```python
from build123d import *

# Parameters (mm, degrees)
F1_DEPTH    = 2
F3_DEPTH    = 13
F2_W        = 100
F2_H        = 2
F4_DEPTH    = 25
F5_W        = 1.9823738266
F5_H        = 13
F6_DEPTH    = 6
F7_T1_DEPTH = 18.1433659759
F9_DEPTH    = 25


# Not quite as in the source:
# - a fillet or chamfer that OpenCascade refuses, or shapes differently, is made with other operations: its cross-section is extruded or revolved along the edge and cut away or added


with BuildPart() as f1:
    # F0 (on Front) → F1 (new body)
    with BuildSketch(Plane.XZ):
        Polygon((-26.6649637938, 13), (-26.6649637938, 0), (73.3350362062, -8.7488663526), (73.3350362062, 13), align=None)
    extrude(amount=F1_DEPTH)

    # F2 (on face) → F3 (join)
    with BuildSketch(Plane.XZ.offset(2)):
        Polygon((73.3350362062, -6.7412266775), (-26.6649136147, 2.007635285), (-26.6649637938, 0), (73.3350362062, -8.7488663526), align=None)
    extrude(amount=F3_DEPTH)

    # F2 (on face) → F4 (join)
    with BuildSketch(Plane.XZ.offset(2)):
        with Locations((23.3350362062, 12)):
            Rectangle(F2_W, F2_H)
    extrude(amount=F4_DEPTH)

    # F5 (on face) → F6 (join)
    with BuildSketch(Plane(origin=(-0.0282388724, 0, -0.322771789), x_dir=(0.9961946981, 0, -0.0871557427), z_dir=(0.0871557427, 0, 0.9961946981))):
        with Locations((72.6523239577, -8.5)):
            Rectangle(F5_W, F5_H)
    extrude(amount=F6_DEPTH)

    # F7: chamfer of 2 on 1 edges, made by hand

    # F7_s2 → F7_t1 (cut)
    with BuildSketch(Plane.XZ.offset(2)):
        Polygon((73.6836591771, -2.7564478851), (71.8655812665, -0.5897470035), (73.8579706626, -0.764058489), align=None)
    extrude(amount=F7_T1_DEPTH, mode=Mode.SUBTRACT)

    # F8 (on face) → F9 (cut)
    with BuildSketch(Plane(origin=(0, -2, 0), x_dir=(-1, 0, 0), z_dir=(0, 1, 0))):
        Polygon((-73.6836591771, -2.7564478851), (-73.3350362062, -6.7412266775), (-73.3350362062, -2.340975207), align=None)
    extrude(amount=-F9_DEPTH, mode=Mode.SUBTRACT)


solid = f1.part
```
Geometry check sheet. Reference: the model listing, model coordinates, mm. A direction names the side the tool comes from. Give positions to 0.01 mm unless a question says otherwise; leave off trailing zeros. Write each loop counter-clockwise with the first axis right and the second up, starting at its lowest first coordinate (ties: lowest second). Pieces come first, ordered by that corner, then holes.
1) Gauge pin test, flat ends, axial feed: pin 1 (6 mm diameter, centred on x = 43.5, y = -6, fed in from -Z); pin 2 (2 mm diameter, centred on x = -1, z = -0.5, fed in from -Y); pin 3 (1.5 mm diameter, centred on x = -9.5, y = -15, fed in from -Z). Record the tip position at first contact, or that the pin passes through.
2) Access from +Z, -Z, +X, -X, +Y, -Y to the whole of each face (thin tool, end or side, straight path). Record for faces 1 (the flat face through (72.62, -8.41, -1.49)), 2 (the flat face through (23, -13, 13)), 3 (the flat face through (23, -2, 4)).
3) Section check A-A, the plane y = -10.75. Record the boundary of the cut face in (x, z), and give its area (3 significant figures).
4) Section check D-D, the plane y = -21. Record the boundary of the cut face in (x, z), and give its area (3 significant figures).
5) Material ranges on L1, parallel to Z at x = 23.5, y = -25; L2, parallel to Y at x = 53, z = -3.5; L3, parallel to Z at x = 18.5, y = -3.75, recorded low to high.
6) Release check for a two-part mould opening along Z. For faces 4 (the flat face through (23, -14, 11)), 5 (the flat face through (27, -15, -3)), 6 (the flat face through (23.03, -8.41, -2.34)), 7 (the flat face through (22.635, -7.395, -4.313)) record: pulls with the +Z half, pulls with the -Z half, needs draft (parallel to the pull), parting line crosses it, or undercut.
7) Section check C-C, the plane z = 4.75. Record the boundary of the cut face in (x, y), and give its area (3 significant figures).
8) Section check B-B, the plane x = 18.5. Record the boundary of the cut face in (y, z), and give its area (3 significant figures).
Computed:
1. pin 1: stops at z = -6.4
1. pin 2: stops at y = -15
1. pin 3: stops at z = -1.57
2. face 1: +X, -Y
2. face 2: +Z, +X, -X, +Y, -Y
2. face 3: -Y
3. outline: (-26.66, 0) - (73.34, -8.75) - (73.34, -2.34) - (71.88, -0.61) - (71.36, -6.57) - (-26.66, 2.01) - close; (-26.66, 11) - (73.34, 11) - (73.34, 13) - (-26.66, 13) - close
3. area: 410 mm2
4. outline: (-26.66, 11) - (73.34, 11) - (73.34, 13) - (-26.66, 13) - close
4. area: 200 mm2
5. L1: z = 11 to 13
5. L2: y = -2 to 0
5. L3: z = -3.95 to -1.94, 11 to 13
6. face 4: undercut
6. face 5: needs draft
6. face 6: undercut
6. face 7: pulls with the -Z half
7. outline: (-26.66, -2) - (73.34, -2) - (73.34, 0) - (-26.66, 0) - close
7. area: 200 mm2
8. outline: (-27, 11) - (-2, 11) - (-2, -1.94) - (-15, -1.94) - (-15, -3.95) - (0, -3.95) - (0, 13) - (-27, 13) - close
8. area: 110 mm2
